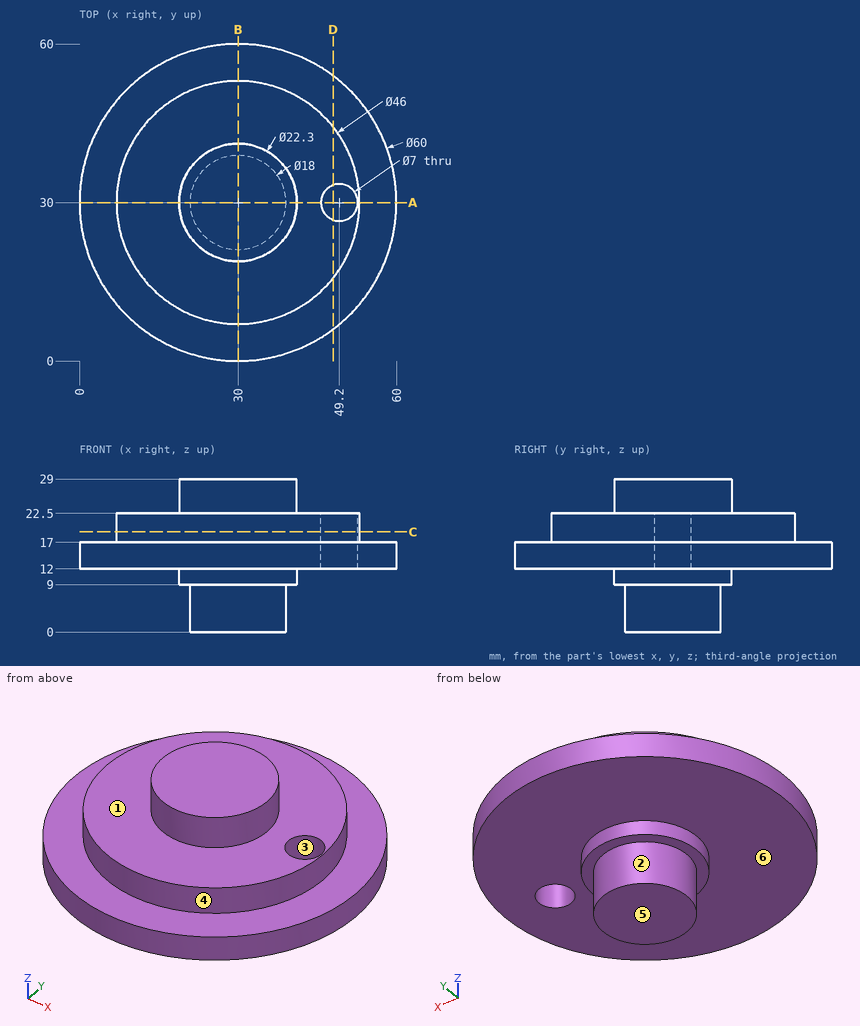
Verification items for this drawing (mm, ordinates from the low corner). A direction names the side the tool comes from. Give positions to 0.01 mm unless a question says otherwise; leave off trailing zeros. Loops run counter-clockwise (first coordinate to the right, second up) from the corner with the lowest first, then second, coordinate; pieces in that order, holes last.
1. Cross-section at B-B on x = 30. Record the cut outline in (y, z), and give its area (3 significant figures).
Derived:
outline: (0, 12) - (18.85, 12) - (18.85, 9) - (21, 9) - (21, 0) - (39, 0) - (39, 9) - (41.15, 9) - (41.15, 12) - (60, 12) - (60, 17) - (53, 17) - (53, 22.5) - (41.15, 22.5) - (41.15, 29) - (18.85, 29) - (18.85, 22.5) - (7, 22.5) - (7, 17) - (0, 17) - close
area: 927 mm2
2. Material ranges on probe 1 along Z at (x, y) = (24.5, 49); probe 2 along Y at (x, z) = (48, 17.75); probe 3 along Z at (x, y) = (28, 56), recorded low to high.
Derived:
probe 1: z = 12 to 22.5
probe 2: y = 15.68 to 26.71, 33.29 to 44.32
probe 3: z = 12 to 17
3. Cross-section at C-C on z = 19. Record the cut outline in (x, y), and give its area (3 significant figures).
Derived:
outline: circle Ø46 at (30, 30); hole circle Ø7 at (49.2, 30)
area: 1,620 mm2
4. Go/stop test with flat-tipped pins: P1, Ø10, axis at x = 10, y = 9.5, coming from the +Z side; P2, Ø8, axis at x = 7.5, y = 18, coming from the +Z side; P3, Ø4, axis at y = 11.5, z = 14, coming from the -X side (1 decimal); P4, Ø18, axis at x = 28, y = 27, coming from the -Z side. Record where each tip stops, or that it passes through.
Derived:
P1: stops at z = 17
P2: stops at z = 22.5
P3: stops at x = 4.9
P4: stops at z = 0
5. Release check for a two-part mould opening along Y. For the marked faces 1, 2 and 3 record: +Y half, -Y half, draft (parallel to the pull), parting line (faces both ways), or undercut.
Derived:
face 1: draft
face 2: parting line
face 3: undercut
6. Cross-section at D-D on x = 48. Record the cut outline in (y, z).
Derived:
outline: (6, 12) - (26.71, 12) - (26.71, 22.5) - (15.68, 22.5) - (15.68, 17) - (6, 17) - close; (33.29, 12) - (54, 12) - (54, 17) - (44.32, 17) - (44.32, 22.5) - (33.29, 22.5) - close
7. Cross-section at A-A on y = 30. Record the cut outline in (x, z), and give its area (3 significant figures).
Derived:
outline: (0, 12) - (18.85, 12) - (18.85, 9) - (21, 9) - (21, 0) - (39, 0) - (39, 9) - (41.15, 9) - (41.15, 12) - (45.7, 12) - (45.7, 22.5) - (41.15, 22.5) - (41.15, 29) - (18.85, 29) - (18.85, 22.5) - (7, 22.5) - (7, 17) - (0, 17) - close; (52.7, 12) - (60, 12) - (60, 17) - (53, 17) - (53, 22.5) - (52.7, 22.5) - close
area: 853 mm2
8. Tool access check on the marked faces 4, 5 and 6. Record the directions out of +Z, -Z, +X, -X, +Y, -Y that give a thin tool (end or side, any length) a straight path to the whole face; none if there is none.
Derived:
face 4: +Z
face 5: -Z, +X, -X, +Y, -Y
face 6: -Z
